```python
from build123d import *

# Parameters (mm, degrees)
F1_DEPTH = 7.5
F2_DEPTH = 5.25


# Not quite as in the source:
# - ends of sketch curves that miss each other by under 0.0002 mm in the source are joined


with BuildPart() as f1:
    # F0 (on Front) → F1 (new body, symmetric)
    with BuildSketch(Plane.XZ):
        with BuildLine():
            ThreePointArc((-11.0043239024, 7.1529938994), (-0.6435162461, 7.0398408721), (9.3939724206, 4.4692455787))
            Line((9.3939724206, 4.4692455787), (10.7793952497, 8.0129774852))
            Line((10.7793952497, 8.0129774852), (-11.4156674583, 10.8236569963))
            Line((-11.4156674583, 10.8236569963), (-11.0043239024, 7.1529938994))
        make_face()
        with BuildLine():
            Line((4.1502654463, -8.9435067945), (9.39397455, 4.4692447462))
            ThreePointArc((9.39397455, 4.4692447462), (-0.6435162461, 7.0398408721), (-11.0043239024, 7.1529938994))
            Line((-11.0043239024, 7.1529938994), (-9.3998677417, -7.1645337772))
            ThreePointArc((-9.3998677417, -7.1645337772), (-3.3213281789, -13.3593367926), (4.1502654463, -8.9435067945))
        make_face()
        with BuildLine():
            ThreePointArc((-3.3084953622, -0.8006877888), (-1.4860286023, 0.5975869129), (-0.0877539006, -1.2248798469))
            Line((-0.0877539006, -1.2248798469), (-0.7947424255, -6.5927825509))
            ThreePointArc((-0.7947424255, -6.5927825509), (-2.6172092627, -7.9910572424), (-4.0154839644, -6.1685904826))
            Line((-4.0154839644, -6.1685904826), (-3.3084953622, -0.8006877888))
        make_face(mode=Mode.SUBTRACT)
    extrude(amount=F1_DEPTH, both=True)

    # F0 (on Front) → F2 (cut, symmetric)
    with BuildSketch(Plane.XZ):
        with BuildLine():
            Line((4.1502654463, -8.9435067945), (9.39397455, 4.4692447462))
            ThreePointArc((9.39397455, 4.4692447462), (-0.6435162461, 7.0398408721), (-11.0043239024, 7.1529938994))
            Line((-11.0043239024, 7.1529938994), (-9.3998677417, -7.1645337772))
            ThreePointArc((-9.3998677417, -7.1645337772), (-3.3213281789, -13.3593367926), (4.1502654463, -8.9435067945))
        make_face()
        with BuildLine():
            ThreePointArc((-3.3084953622, -0.8006877888), (-1.4860286023, 0.5975869129), (-0.0877539006, -1.2248798469))
            Line((-0.0877539006, -1.2248798469), (-0.7947424255, -6.5927825509))
            ThreePointArc((-0.7947424255, -6.5927825509), (-2.6172092627, -7.9910572424), (-4.0154839644, -6.1685904826))
            Line((-4.0154839644, -6.1685904826), (-3.3084953622, -0.8006877888))
        make_face(mode=Mode.SUBTRACT)
    extrude(amount=F2_DEPTH, both=True, mode=Mode.SUBTRACT)


solid = f1.part
```
Geometry check sheet. Reference: the model listing, model coordinates, mm. A direction names the side the tool comes from. Coordinates: 2 decimals unless noted, no trailing zeros. Order: outer loops, then holes, each group sorted by start corner. A loop starts at its lowest first (then second) coordinate and runs counter-clockwise, first axis right, second up. Notation, with made-up numbers: (69, 71) - (123, 71) arc R3 ccw to (123, 75) - close; hole circle Ø4 at (69, 75). An arc over 180 degrees is marked (long way). Answer in a Markdown table with one row per item. Add a question column.
1. Material ranges on L1, parallel to Y at x = -5, z = 6.75; L2, parallel to X at y = 5.5, z = -6.75; L3, parallel to Z at x = 2, y = 1, recorded low to high. Write a range as [from, to].
2. Section check B-B (x = -1.25). Enter the section's corners in (y, z).
3. Section check C-C (z = 1.5). Enter the section's corners in (x, y), plus the area to 3 significant figures.
4. Section check A-A (z = -2.25). Enter the section's corners in (x, y).
5. Access from +Z, -Z, +X, -X, +Y, -Y to the whole of each face (thin tool, end or side, straight path). Record for faces 1 (the face through (-0.5, -0.07, 7.02)), 2 (the face through (-3.667, 6.359, -3.522)), 3 (the face through (6.735, -6.391, -2.331)).
6. Section check D-D (x = -4.5). Enter the section's corners in (y, z).
7. Draft check along Z on faces 4 (the face through (-0.16, -0.11, 9.4)), 5 (the face through (-3.45, -6.39, -13.34)), 6 (the face through (-0.436, -6.391, -3.871)). Enter one of: +Z half, -Z half, draft (parallel to the pull), parting line (faces both ways), or undercut.
8. Gauge pin test, flat ends, axial feed: pin 1 Ø1.5 at (x, y) = (-7.5, 0.5) entering from +Z; pin 2 Ø4 at (x, y) = (1, 3.5) entering from -Z; pin 3 Ø1.5 at (y, z) = (3, 1) entering from +X; pin 4 Ø8 at (y, z) = (-5, -4.5) entering from +X. Record the tip position at first contact, or that the pin passes through.
Data:
| question | item | result |
|---|---|---|
| 1 | L1 | y = [-7.5, -5.25], [5.25, 7.5] |
| 1 | L2 | x = [-9.45, -3.99], [-0.82, 5.01] |
| 1 | L3 | z = [6.61, 9.12] |
| 2 | outline | (-7.5, -13.32) - (-5.25, -13.32) - (-5.25, -7.52) - (-7.5, -7.52) - close; (-7.5, 0.55) - (-5.25, 0.55) - (-5.25, 7.12) - (5.25, 7.12) - (5.25, 0.55) - (7.5, 0.55) - (7.5, 9.54) - (-7.5, 9.54) - close; (5.25, -13.32) - (7.5, -13.32) - (7.5, -7.52) - (5.25, -7.52) - close |
| 3 | outline | (-10.37, -7.5) - (8.23, -7.5) - (8.23, -5.25) - (-10.37, -5.25) - close; (-10.37, 5.25) - (8.23, 5.25) - (8.23, 7.5) - (-10.37, 7.5) - close |
| 3 | area | 83.7 mm² |
| 4 | outline | (-9.95, -7.5) - (-3.5, -7.5) - (-3.5, -5.25) - (-9.95, -5.25) - close; (-9.95, 5.25) - (-3.5, 5.25) - (-3.5, 7.5) - (-9.95, 7.5) - close; (-0.22, -7.5) - (6.77, -7.5) - (6.77, -5.25) - (-0.22, -5.25) - close; (-0.22, 5.25) - (6.77, 5.25) - (6.77, 7.5) - (-0.22, 7.5) - close |
| 5 | face 1 | -Z |
| 5 | face 2 | +Y, -Y |
| 5 | face 3 | -Z, +X, +Y, -Y |
| 6 | outline | (-7.5, -13.1) - (-5.25, -13.1) - (-5.25, 7.37) - (5.25, 7.37) - (5.25, -13.1) - (7.5, -13.1) - (7.5, 9.95) - (-7.5, 9.95) - close |
| 7 | face 4 | +Z half |
| 7 | face 5 | -Z half |
| 7 | face 6 | undercut |
| 8 | pin 1 | stops at z = 10.42 |
| 8 | pin 2 | stops at z = -12.98 |
| 8 | pin 3 | passes through |
| 8 | pin 4 | stops at x = 7.45 |
